Can you work these out from the drawing? Everything is in mm from the part's minimum corner. A direction names the side the tool comes from. Round coordinates to 2 decimals unless told otherwise and drop trailing zeros. Loops run counter-clockwise (first coordinate to the right, second up) from the corner with the lowest first, then second, coordinate; pieces in that order, holes last. Notation, with made-up numbers: (57.25, 69.25) -> (84.25, 69.25) arc R30 ccw to (84.25, 102.25) -> close; hole circle Ø11 at (-1, 38.5). An arc over 180 degrees is marked (long way). One line per item, written item: value.
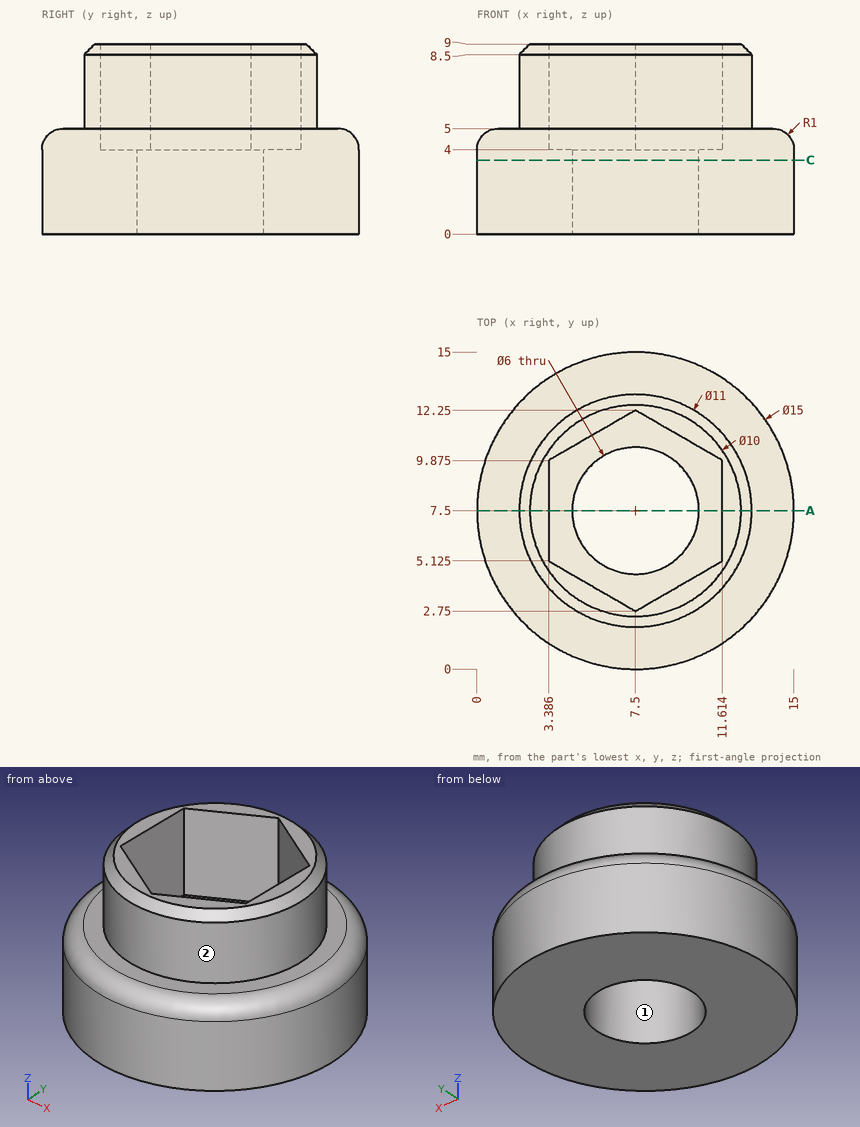
(1) Please list where these lines run through material, in increasing order: L1, parallel to Y at x = 7.5, z = 2.8; L2, parallel to Z at x = 9.25, y = 10; L3, parallel to X at y = 10, z = 8.75 (1 decimal).
Results below:
L1: y = 0 to 4.5, 10.5 to 15
L2: z = 0 to 4
L3: x = 2.9 to 3.6, 11.4 to 12.1
(2) For pin 1 Ø1.5 at (y, z) = (2.5, 4) entering from +X; pin 2 Ø2.5 at (y, z) = (8.5, 7.5) entering from +X; pin 3 Ø3 at (y, z) = (10.5, 5.5) entering from -X, each with a flat end and sliding along its axis, tell me the tip position at first contact or that it passes through.
Results below:
pin 1: stops at x = 13.68
pin 2: stops at x = 13
pin 3: stops at x = 0.35
(3) Imagine slicing it at C-C on z = 3.5. Write out the boundary of the cut face in (x, y).
Results below:
outline: circle Ø15 at (7.5, 7.5); hole circle Ø6 at (7.5, 7.5)
(4) On a 3-axis mill with a long thin cutter (end or side, diameter ignored), from which of +Z, -Z, +X, -X, +Y, -Y can I reach the whole of each face in a straight line? I mean the marked faces 1 and 2. Say none if no direction works.
Results below:
face 1: +Z, -Z
face 2: +Z
(5) Imagine slicing it at A-A on y = 7.5. Write out the boundary of the cut face in (x, z).
Results below:
outline: (0, 0) -> (4.5, 0) -> (4.5, 4) -> (3.39, 4) -> (3.39, 9) -> (2.5, 9) -> (2, 8.5) -> (2, 5) -> (1, 5) arc R1 ccw to (0, 4) -> close; (10.5, 0) -> (15, 0) -> (15, 4) arc R1 ccw to (14, 5) -> (13, 5) -> (13, 8.5) -> (12.5, 9) -> (11.61, 9) -> (11.61, 4) -> (10.5, 4) -> close
